Design review of the part built by this model. Coordinates are the model's own, in mm. Face numbers are marked on the shaded views. Coordinates: 2 decimals unless noted, no trailing zeros. Write each loop counter-clockwise with the first axis right and the second up, starting at its lowest first coordinate (ties: lowest second). Pieces come first, ordered by that corner, then holes. Notation, with made-up numbers: M 19,-4 L 30,-4 A18 cw 30,10 Z; hole C 85.5,-33 d5. An arc over 180 degrees is marked long. Write item = value, one per line.
```python
from build123d import *

# Parameters (mm, degrees)
SKETCH1_W      = 71.6
SKETCH1_H      = 2.9
EXTRUDE1_DEPTH = 3.175


with BuildPart() as part:
    # Sketch1 → Extrude1 (new body)
    with BuildSketch(Plane.XY):
        Polygon((90.427144536, 6.036016451), (90.427144536, 13.036016451), (84.077144536, 13.036016451), (84.077144536, 20.586016451), (75.237144536, 20.586016451), (75.237144536, 19.336016451), (72.987144536, 19.336016451), (72.987144536, 20.586016451), (69.327144536, 20.586016451), (69.327144536, 23.486016451), (72.987144536, 23.486016451), (72.987144536, 24.736016451), (75.237144536, 24.736016451), (75.237144536, 23.486016451), (84.077144536, 23.486016451), (84.077144536, 31.036016451), (90.427144536, 31.036016451), (90.427144536, 38.036016451), (-11.172855464, 38.036016451), (-11.172855464, 31.036016451), (-4.822855464, 31.036016451), (-4.822855464, 23.486016451), (4.017144536, 23.486016451), (4.017144536, 24.736016451), (6.267144536, 24.736016451), (6.267144536, 23.486016451), (9.927144536, 23.486016451), (9.927144536, 20.586016451), (6.267144536, 20.586016451), (6.267144536, 19.336016451), (4.017144536, 19.336016451), (4.017144536, 20.586016451), (-4.822855464, 20.586016451), (-4.822855464, 13.036016451), (-11.172855464, 13.036016451), (-11.172855464, 6.036016451), align=None)
        with Locations((39.627144536, 12.486016451)):
            Rectangle(SKETCH1_W, SKETCH1_H, mode=Mode.SUBTRACT)
    extrude(amount=EXTRUDE1_DEPTH)


solid = part.part
```
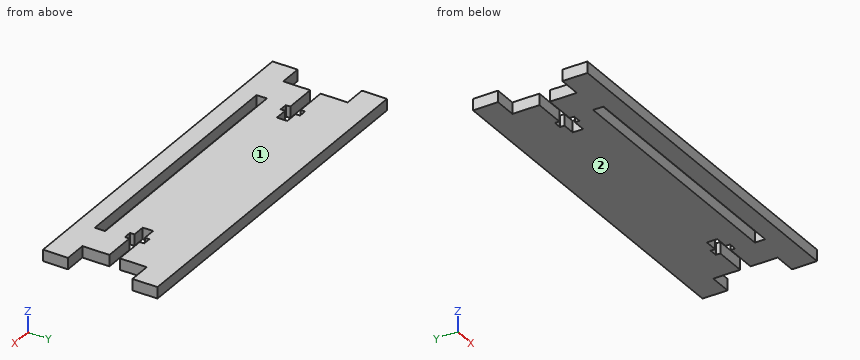
Q1. The part is to be moulded in two halves that separate along Z. For the marked faces 1 and 2, say which applies: +Z half, -Z half, draft (parallel to the pull), parting line (faces both ways), or undercut.
Check result:
face_1 = +Z half
face_2 = -Z half
Q2. For P1, Ø1, axis at y = 16, z = 2, coming from the +X side; P2, Ø0.6, axis at y = 20, z = 1.5, coming from the -X side, all flat-tipped, find the tip position at first contact; note any pin that passes through.
Check result:
P1 = 84.08
P2 = -4.82
Q3. Consider section B-B, the plane x = 71. State the section outline as (y, z) points (3 decimals).
Check result:
outline = M 6.036,0 L 11.036,0 L 11.036,3.175 L 6.036,3.175 Z; M 13.936,0 L 20.586,0 L 20.586,3.175 L 13.936,3.175 Z; M 23.486,0 L 38.036,0 L 38.036,3.175 L 23.486,3.175 Z
Q4. Consider section A-A, the plane x = 17.5. State the section outline as (y, z) points (3 decimals).
Check result:
outline = M 6.036,0 L 11.036,0 L 11.036,3.175 L 6.036,3.175 Z; M 13.936,0 L 38.036,0 L 38.036,3.175 L 13.936,3.175 Z
Q5. Consider section C-C, the plane y = 28. State the section outline as (x, z) points (3 decimals), and give its area (3 significant figures).
Check result:
outline = M -4.823,0 L 84.077,0 L 84.077,3.175 L -4.823,3.175 Z
area = 282 mm²
Q6. Wall thickness on line 1 (X direction, y = 24, z = 0.3); line 2 (Y direction, x = 14.5, z = 0.55); line 3 (Y direction, x = 0, z = 1.25): over which ranges is each line inside the solid? List them lowest first.
Check result:
line_1 = -4.82 to 4.02, 6.27 to 72.99, 75.24 to 84.08
line_2 = 6.04 to 11.04, 13.94 to 38.04
line_3 = 6.04 to 20.59, 23.49 to 38.04
